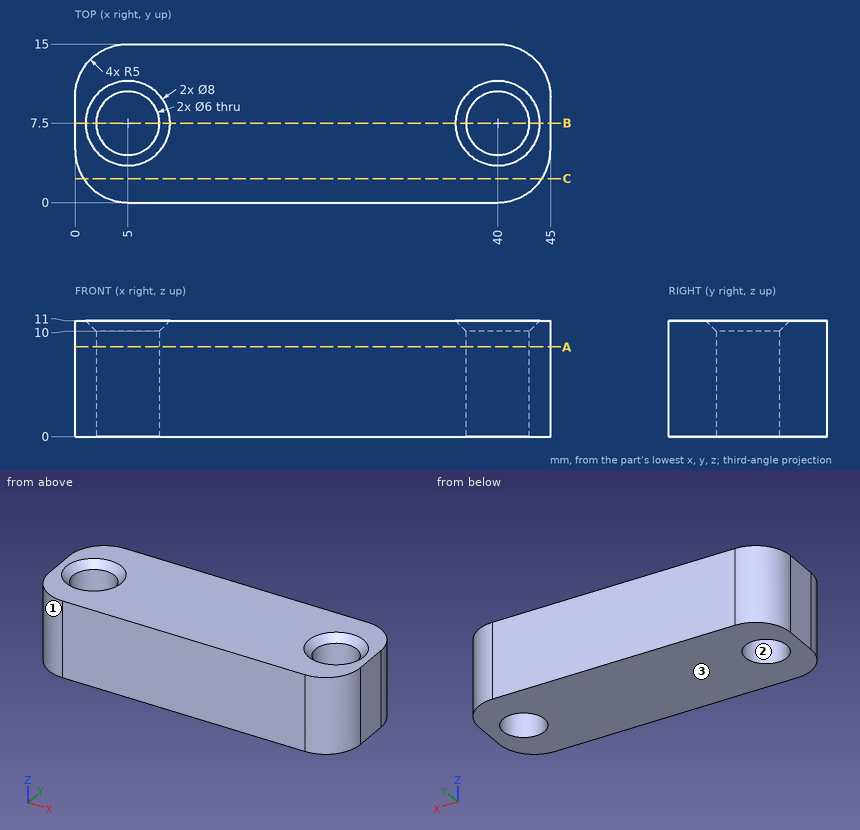
Study the drawing (mm; zero at the part's minimum x, y, z) and answer. Round coordinates to 2 decimals unless told otherwise and drop trailing zeros. Loops run counter-clockwise (first coordinate to the right, second up) from the corner with the lowest first, then second, coordinate; pieces in that order, holes last.
Q1. Section C-C, the plane y = 2.25 is taken. Determine the outline of the cut face in (x, z).
Q2. Section A-A, the plane z = 8.5 is taken. Determine the outline of the cut face in (x, y).
Q3. Find the intervals of material crossed by line 1 (X direction, y = 7.25, z = 7); line 2 (Y direction, x = 40, z = 7); line 3 (X direction, y = 5.25, z = 3.5), in increasing order.
Q4. For a pull along Y with two mould halves and no side action, classify the marked faces 1, 2 and 3 as released by +Y, released by -Y, zero draft, split by the parting line, or undercut.
Q5. Section B-B, the plane y = 7.5 is taken. Determine the outline of the cut face in (x, z), then the cut area to 3 significant figures.
Completed:
1. outline: (0.82, 0) - (44.18, 0) - (44.18, 11) - (0.82, 11) - close
2. outline: (0, 5) arc R5 ccw to (5, 0) - (40, 0) arc R5 ccw to (45, 5) - (45, 10) arc R5 ccw to (40, 15) - (5, 15) arc R5 ccw to (0, 10) - close; hole circle Ø6 at (5, 7.5); hole circle Ø6 at (40, 7.5)
3. line 1: x = 0 to 2.01, 7.99 to 37.01, 42.99 to 45
3. line 2: y = 0 to 4.5, 10.5 to 15
3. line 3: x = 0 to 3.02, 6.98 to 38.02, 41.98 to 45
4. face 1: released by -Y
4. face 2: undercut
4. face 3: zero draft
5. outline: (0, 0) - (2, 0) - (2, 10) - (1, 11) - (0, 11) - close; (8, 0) - (37, 0) - (37, 10) - (36, 11) - (9, 11) - (8, 10) - close; (43, 0) - (45, 0) - (45, 11) - (44, 11) - (43, 10) - close
5. area: 361 mm2
